Input: part model. Units: mm. Frame: model coordinates. Round coordinates to 2 decimals unless told otherwise and drop trailing zeros. Loops run counter-clockwise (first coordinate to the right, second up) from the corner with the lowest first, then second, coordinate; pieces in that order, holes last. Notation, with made-up numbers: (42, -38.5) -> (66, -38.5) arc R30 cw to (66, -7.5) -> close; hole circle Ø6 at (-29, 69). An arc over 180 degrees is marked (long way). Answer as a JSON object with one key per item and string values. Group by question number.
Item 1: Section query C-C on y = 1. Return loops of the section in (x, z).
Item 2: Material intervals for line 1 (Y direction, x = 40.5, z = 961); line 2 (Y direction, x = 39.5, z = 550.5); line 3 (X direction, y = 1, z = 1984.5), sorted ascending. Write a range as [from, to].
Item 3: Section query B-B on z = 1518. Return loops of the section in (x, y).
Item 4: Pin query (flat end, axial travel): pin 1 (1.5 mm diameter, centred on y = -26.5, z = 866.5, fed in from +X); pin 2 (6 mm diameter, centred on y = 17.5, z = 1589.5, fed in from +X). Return the tip coordinate at first contact, or that it passes through.
Item 5: Section query A-A on x = 32.5. Return loops of the section in (y, z).
Item 6: Draft query along Y for faces 1 (the flat face through (4.07, 0, 1186)), 2 (the flat face through (21, -40, 1186)), 3 (the flat face through (3, 0, 2365)). Return one class per face: released by +Y, released by -Y, zero draft, split by the parting line, or undercut.
Autodesk Inventor part; units mm, degrees
ref_plane "Начальная плоскость" through (0, 0, 40) normal (0, 0, 1) x (1, 0, 0)
ref_plane "Конечная плоскость" through (0, 0, 2365) normal (0, 0, 1) x (1, 0, 0)
ref_plane "РабПлоскость4" through (-1.43, 1200, 40) normal (0, 0, -1) x (-1, 0, 0)
ref_plane "Начальная плоскость" through (0, 0, 40) normal (0, 0, 1) x (1, 0, 0)
ref_plane "Конечная плоскость" through (0, 0, 2365) normal (0, 0, 1) x (1, 0, 0)
sketch "Эскиз" plane through (0, 0, 0) normal (0, 0, 1) x (1, 0, 0)
  line L0 (-1.43, 0) -> (-1.43, 40)
  line L1 (-1.43, 40) -> (43.57, 40)
  line L2 (43.57, 40) -> (43.57, 38.1774)
  line L3 (39.9881, 34.1993) -> (11.2338, 31.1771)
  line L4 (4.07, 23.221) -> (4.07, 0)
  line L5 (4.07, 0) -> (-1.43, 0) construction
  line L6 (23.82, 40) -> (23.82, 32.5) construction
  line L7 (43.57, 34.5758) -> (43.57, 32.5) construction
  line L8 (43.57, 32.5) -> (23.82, 32.5) construction
  line L9 (0, 15) -> (0, -27) construction
  line L10 (-5.539, 0) -> (16.0067, 0) construction
  line L11 (-1.43, 0) -> (-1.43, -40)
  line L12 (-1.43, -40) -> (43.57, -40)
  line L13 (43.57, -40) -> (43.57, -38.1774)
  line L14 (39.9881, -34.1993) -> (11.2338, -31.1771)
  line L15 (4.07, -23.221) -> (4.07, 0)
  arc A0 (11.2338, 31.1771) -> (4.07, 23.221) centre (12.07, 23.221) ccw
  arc A1 (4.07, -23.221) -> (11.2338, -31.1771) centre (12.07, -23.221) ccw
  arc A2 (39.9881, 34.1993) -> (43.57, 38.1774) centre (39.57, 38.1774) ccw
  arc A3 (43.57, -38.1774) -> (39.9881, -34.1993) centre (39.57, -38.1774) ccw
  line L16 (0, 56) -> (0, -56) construction
  line L17 (-15.5135, 0) -> (54.308, 0) construction
  point P0 (4.07, 30.4242)
  point P1 (43.57, -34.5758)
  point P2 (4.07, -30.4242)
  point P3 (23.82, -40)
  point P4 (23.82, -32.5)
  dimension "d0" = 5.5
  dimension "d1" = 40
  dimension "d2" = 45
  dimension "d3" = 7.5
  dimension "d4" = 19.75
  dimension "d5" = 2.0758
  dimension "d23" = 8
  dimension "d24" = 4
  dimension "d25" = 1.43
extrude "Тело" add sketch "Эскиз" along normal up to surface (2325 mm away) from surface at 40
sketch "Sketch3" plane through (0, 0, 0) normal (0, 0, 1) x (1, 0, 0)
  line L0 (0, 0) -> (10, 0)
ref_plane "Work Plane3" through (0, 0, 0) normal (0, -1, 0) x (1, 0, 0)
sketch "Sketch4" plane through (0, 0, 0) normal (0, -1, 0) x (1, 0, 0)
  line L0 (-2, 40) -> (12, 40)
  line L1 (-2, 2365) -> (12, 2365)
  dimension "d29" = 2325
ref_plane "РабПлоскость4" through (-1.43, 1200, 40) normal (0, 0, -1) x (-1, 0, 0)
split "Разделение1" plane through (-1.43, 1200, 40) removes the side toward (0, 0, -1)
ref_plane "РабПлоскость5" through (-1.43, -520, 2365) normal (0, 0, 1) x (1, 0, 0)
split "Разделение2" plane through (-1.43, -520, 2365) removes the side toward (0, 0, 1)
equation "\"d0\" = G_T"
equation "\"d1\" = 0.5 * G_H"
equation "\"d2\" = G_W"
equation "\"d3\" = G_T1"
equation "\"d4\" = G_C"
equation "\"d23\" = G_IR"
equation "\"d24\" = G_ER"
equation "\"d25\" = ex"
equation "\"d6\" = G_L"
equation "\"G_W\" = 45"
equation "\"G_T\" = 5.5"
equation "\"G_T1\" = 7.5"
equation "\"G_NG\" = 0.105104"
equation "\"G_ER\" = 4"
equation "\"G_IR\" = 8"
equation "\"G_C\" = 19.75"
equation "\"G_L\" = d29"
equation "\"ex\" = 1.43"
equation "\"d27\" = G_OFFSET_END + B_L"
equation "\"B_L\" = 2405"
properties part number "ISO 657/11 - CH 80 x 8 - 2325" material "Сталь, мягкая"
Solved:
{
 "1": {"outline": "(-1.43, 40) -> (4.07, 40) -> (4.07, 2365) -> (-1.43, 2365) -> close"},
 "2": {"line 1": "[-40, -34.29], [34.29, 40]", "line 2": "[-40, -34.15], [34.15, 40]", "line 3": "[-1.43, 4.07]"},
 "3": {"outline": "(-1.43, -40) -> (43.57, -40) -> (43.57, -38.18) arc R4 ccw to (39.99, -34.2) -> (11.23, -31.18) arc R8 cw to (4.07, -23.22) -> (4.07, 23.22) arc R8 cw to (11.23, 31.18) -> (39.99, 34.2) arc R4 ccw to (43.57, 38.18) -> (43.57, 40) -> (-1.43, 40) -> close"},
 "4": {"pin 1": "x = 5.16", "pin 2": "x = 4.07"},
 "5": {"outline": "(-40, 40) -> (-33.41, 40) -> (-33.41, 2365) -> (-40, 2365) -> close; (33.41, 40) -> (40, 40) -> (40, 2365) -> (33.41, 2365) -> close"},
 "6": {"face 1": "undercut", "face 2": "released by -Y", "face 3": "zero draft"}
}
